The model under review builds one solid part; all positions refer to its coordinate system, in mm. A direction names the side the tool comes from. Coordinates: 2 decimals unless noted, no trailing zeros. Answer in a Markdown table with one row per item. Add a question column.
(1) We need section A-A on x = 0. Give the number of separate pieces and of enclosed holes in the cut face, plus the area to 3 significant figures.
(2) For line 1 along X through (y, z) = (0.25, -0.75); line 2 along X through (y, z) = (1.45, 0.75); line 3 along X through (y, z) = (2.05, 0), list the stretches that pass through material, from the lowest coordinate up.
(3) Mouldability with a two-part tool opening along Z and no side actions: class faces 3 (the cylindrical face through (-11.3, 0.5, -0.6)), 4 (the flat face through (0, 0, 0)) as +Z half, -Z half, draft (parallel to the pull), parting line (faces both ways), or undercut.
(4) For P1, Ø4.5, axis at x = 11.5, z = -0.5, coming from the +Y side; P2, Ø2.5, axis at x = 10.5, z = 0, coming from the -Y side; P3, Ø1.5, axis at x = 3.5, y = 3, coming from the -Z side; P4, Ø2.5, axis at x = -10.5, z = 0, coming from the +Y side, all flat-tipped, find the tip position at first contact; note any pin that passes through.
(5) Machinability: for faces 1 (the cylindrical face through (9.7, 0.5, -0.6)), 2 (the cylindrical face through (-8.4, 1.84, -0.09)), which of the approach directions +Z, -Z, +X, -X, +Y, -Y give a long, thin tool a straight path to every point of the face, cutting with its end or side? Answer none if there is none.
from build123d import *

# Parameters (mm, degrees)
SKETCH2_W               = 50.634745493
SKETCH2_H               = 13.07277583
CUT_EXTRUDE1_DEPTH      = 5.0000001
CUT_EXTRUDE1_DEPTH_BACK = 5.0000001
SKETCH3_R               = 1
CUT_EXTRUDE2_DEPTH      = 5.0000001
SKETCH4_R               = 2.1
CUT_EXTRUDE3_DEPTH      = 4.0000001
SKETCH5_R               = 1.5
CUT_EXTRUDE4_DEPTH      = 5.0000001


with BuildPart() as part:
    # Sketch1 → Revolve1 (revolve)
    with BuildSketch(Plane.XY):
        with BuildLine():
            Line((-14, 0), (14, 0))
            add(Edge.make_bspline(
                [(14, 0), (14, 4), (0, 4), (-14, 4), (-14, 0)],
                knots=[0, 0, 0, 1.570796327, 1.570796327, 3.141592654, 3.141592654, 3.141592654], degree=2, weights=[1, 0.707106781, 1, 0.707106781, 1]))
        make_face()
    revolve(axis=Axis((-14, 0, 0), (1, 0, 0)))

    # Sketch2 → Cut-Extrude1 (cut, two sides)
    with BuildSketch(Plane.XY) as cut_extrude1_sk:
        with Locations((-1.598405816, -6.536387915)):
            Rectangle(SKETCH2_W, SKETCH2_H)
    extrude(amount=CUT_EXTRUDE1_DEPTH, mode=Mode.SUBTRACT)
    extrude(cut_extrude1_sk.sketch, amount=-CUT_EXTRUDE1_DEPTH_BACK, mode=Mode.SUBTRACT)

    # Sketch3 → Cut-Extrude2 (cut, through all)
    with BuildSketch(Plane.XZ):
        with Locations((-10.5, 0)):
            Circle(SKETCH3_R)
        with Locations((10.5, 0)):
            Circle(SKETCH3_R)
    extrude(amount=-CUT_EXTRUDE2_DEPTH, mode=Mode.SUBTRACT)

    # Sketch4 → Cut-Extrude3 (cut, through all)
    with BuildSketch(Plane(origin=(0, 1, 0), x_dir=(-1, 0, 0), z_dir=(0, -1, 0))):
        with Locations((10.5, 0)):
            Circle(SKETCH4_R)
        with Locations((-10.5, 0)):
            Circle(SKETCH4_R)
    extrude(amount=-CUT_EXTRUDE3_DEPTH, mode=Mode.SUBTRACT)

    # Sketch5 → Cut-Extrude4 (cut, through all)
    with BuildSketch(Plane.XZ):
        with Locations((0, 2)):
            Circle(SKETCH5_R)
        with Locations((0, -2)):
            Circle(SKETCH5_R)
    extrude(amount=-CUT_EXTRUDE4_DEPTH, mode=Mode.SUBTRACT)


solid = part.part
Outcome:
| question | item | result |
|---|---|---|
| 1 | separate pieces | 3 |
| 1 | enclosed holes | 0 |
| 1 | area | 5.30 mm² |
| 2 | line 1 | -13.72 to -11.16, -9.84 to -0.83, 0.83 to 9.84, 11.16 to 13.72 |
| 2 | line 2 | -12.78 to -12.46, -8.54 to -0.83, 0.83 to 8.54, 12.46 to 12.78 |
| 2 | line 3 | -8.4 to 8.4 |
| 3 | face 3 | undercut |
| 3 | face 4 | draft |
| 4 | P1 | y = 2.05 |
| 4 | P2 | y = 0 |
| 4 | P3 | z = -3.16 |
| 4 | P4 | y = 1 |
| 5 | face 1 | +Y, -Y |
| 5 | face 2 | +Y |
